The model under review builds one solid part; all positions refer to its coordinate system, in mm. A direction names the side the tool comes from. Round coordinates to 2 decimals unless told otherwise and drop trailing zeros. Write each loop counter-clockwise with the first axis right and the second up, starting at its lowest first coordinate (ties: lowest second). Pieces come first, ordered by that corner, then holes.
Item 1: Add section D-D (x = 8). Give the boundary of the cut face in (y, z).
Item 2: Draft analysis for pull direction Z (two halves, no side actions). For faces 4 (the face through (20, 17, 0)), 5 (the face through (37.5, 31, -56)), 6 (the face through (38, 2, -59)), 7 (the face through (25.85, 5.28, -2.54)), state which applies: +Z half, -Z half, draft (parallel to the pull), parting line (faces both ways), or undercut.
Item 3: Add section C-C (y = 6). Give the boundary of the cut face in (x, z), plus the area to 4 significant figures.
Item 4: To check wall thickness, follow L1, parallel to X at y = 27, z = -2; L2, parallel to Z at x = 37, y = 27.5; L3, parallel to X at y = 7, z = -24. State the ranges of each line that lie inside material, in increasing order.
Item 5: Add section B-B (x = 36). Give the boundary of the cut face in (y, z), plus the area to 3 significant figures.
Item 6: Clearance check with flat-ended pins moving along their axes: pin 1 Ø6.5 at (y, z) = (29, -54) entering from -X; pin 2 Ø17.5 at (x, y) = (24, 22) entering from -Z. State where each tip first meets the part, or that it passes through.
Item 7: Machinability: for faces 1 (the face through (37, 17, -60)), 2 (the face through (38.768, 30.201, -57.815)), 3 (the face through (35, 17, -32)), which of the approach directions +Z, -Z, +X, -X, +Y, -Y give a long, thin tool a straight path to every point of the face, cutting with its end or side? Answer none if there is none.
Item 8: Add section A-A (z = -31). Give the boundary of the cut face in (x, y), plus the area to 4 significant figures.
```python
from build123d import *

# Parameters (mm, degrees)
BOSS_EXTRUDE1_DEPTH = 35
FILLET1_R           = 5
SKETCH2_R           = 2.5
CUT_EXTRUDE1_DEPTH  = 6
SKETCH3_R           = 2.5
CUT_EXTRUDE3_DEPTH  = 6
SKETCH5_R           = 4
CUT_EXTRUDE5_DEPTH  = 2.5


with BuildPart() as part:
    # Sketch1 → Boss-Extrude1 (new body)
    with BuildSketch(Plane(origin=(0, 0, 0), x_dir=(1, 0, 0), z_dir=(0, 1, 0))):
        Polygon((0, 0), (0, 5), (35, 5), (35, 60), (40, 60), (40, 0), align=None)
    extrude(amount=BOSS_EXTRUDE1_DEPTH)

    # Fillet1
    fillet1_edges = [part.edges().sort_by_distance(p)[0] for p in [
        (37.5, 35, -60),
        (37.5, 0, -60),
    ]]
    fillet(fillet1_edges, radius=FILLET1_R)

    # Sketch2 → Cut-Extrude1 (cut, through all)
    with BuildSketch(Plane(origin=(0, 0, -5), x_dir=(-1, 0, 0), z_dir=(0, 0, -1))):
        with Locations((-27.000416448, 27.5)):
            Circle(SKETCH2_R)
        with Locations((-8.85118862, 27.5)):
            Circle(SKETCH2_R)
        with Locations((-27.000416448, 7.5)):
            Circle(SKETCH2_R)
        with Locations((-8.85118862, 7.5)):
            Circle(SKETCH2_R)
    extrude(amount=-CUT_EXTRUDE1_DEPTH, mode=Mode.SUBTRACT)

    # Sketch3 → Cut-Extrude3 (cut, through all)
    with BuildSketch(Plane.ZY.offset(-35)):
        with Locations((-31, 29)):
            Circle(SKETCH3_R)
        with Locations((-54, 6)):
            Circle(SKETCH3_R)
        with Locations((-54, 29)):
            Circle(SKETCH3_R)
        with Locations((-31, 6)):
            Circle(SKETCH3_R)
    extrude(amount=-CUT_EXTRUDE3_DEPTH, mode=Mode.SUBTRACT)

    # Sketch5 → Cut-Extrude5 (cut)
    with BuildSketch(Plane(origin=(40, 0, 0), x_dir=(0, 0, -1), z_dir=(1, 0, 0))):
        with Locations((54, 29)):
            Circle(SKETCH5_R)
        with Locations((31, 6)):
            Circle(SKETCH5_R)
    extrude(amount=-CUT_EXTRUDE5_DEPTH, mode=Mode.SUBTRACT)


solid = part.part
```
Numbers:
1. outline: (0, -5) - (5.15, -5) - (5.15, 0) - (0, 0) - close; (9.85, -5) - (25.15, -5) - (25.15, 0) - (9.85, 0) - close; (29.85, -5) - (35, -5) - (35, 0) - (29.85, 0) - close
2. face 4: +Z half
2. face 5: undercut
2. face 6: -Z half
2. face 7: draft
3. outline: (0, -5) - (6.85, -5) - (6.85, 0) - (0, 0) - close; (10.85, -5) - (25, -5) - (25, 0) - (10.85, 0) - close; (29, -5) - (35, -5) - (35, -28.5) - (37.5, -28.5) - (37.5, -27) - (40, -27) - (40, 0) - (29, 0) - close; (35, -60) - (40, -60) - (40, -56.5) - (35, -56.5) - close; (35, -51.5) - (40, -51.5) - (40, -35) - (37.5, -35) - (37.5, -33.5) - (35, -33.5) - close
3. area: 377.5 mm2
4. L1: x = 0 to 6.4, 11.3 to 24.55, 29.45 to 40
4. L2: z = -60 to -56, -52 to -33, -29 to 0
4. L3: x = 35 to 40
5. outline: (0, -55) arc R5 ccw to (5, -60) - (30, -60) arc R5 ccw to (35, -55) - (35, 0) - (0, 0) - close; hole circle Ø5 at (6, -54); hole circle Ø5 at (6, -31); hole circle Ø5 at (29, -54); hole circle Ø5 at (29, -31)
5. area: 2,010 mm2
6. pin 1: stops at x = 35
6. pin 2: stops at z = -5
7. face 1: -Z, +X, -X, +Y, -Y
7. face 2: +X
7. face 3: -Z, -X, +Y, -Y
8. outline: (35, 0) - (40, 0) - (40, 2) - (37.5, 2) - (37.5, 3.5) - (35, 3.5) - close; (35, 8.5) - (37.5, 8.5) - (37.5, 10) - (40, 10) - (40, 26.5) - (35, 26.5) - close; (35, 31.5) - (40, 31.5) - (40, 35) - (35, 35) - close
8. area: 117.5 mm2
